Here's how the part is built. I have some questions about the finished solid (model axes, mm). A direction names the side the tool comes from. Give positions to 0.01 mm unless a question says otherwise; leave off trailing zeros. Write each loop counter-clockwise with the first axis right and the second up, starting at its lowest first coordinate (ties: lowest second). Pieces come first, ordered by that corner, then holes. Notation, with made-up numbers: (21.5, -24) -> (61.5, -24) arc R15 ccw to (61.5, -5) -> close; hole circle Ø10 at (56, 9.25). An arc over 180 degrees is marked (long way). Answer as CSV lines item,"result". Start each with the question number.
from build123d import *

# Parameters (mm, degrees)
BOX001_W     = 38.1
BOX001_H     = 12.7
BOX001_DEPTH = 50.8
BOX002_W     = 41.3004
BOX002_H     = 15.9004
BOX002_DEPTH = 50.8


with BuildPart() as cube001:
    # Box001 → Box001 (new body)
    with BuildSketch(Plane(origin=(1.6002, 1.6002, 1.6002), x_dir=(1, 0, 0), z_dir=(0, 0, 1))):
        with Locations((19.05, 6.35)):
            Rectangle(BOX001_W, BOX001_H)
    extrude(amount=BOX001_DEPTH)


with BuildPart() as cut:
    # Box002 → Box002 (new body)
    with BuildSketch(Plane.XY):
        with Locations((20.6502, 7.9502)):
            Rectangle(BOX002_W, BOX002_H)
    extrude(amount=BOX002_DEPTH)

    # Cut: cut Cube001
    add(cube001.part, mode=Mode.SUBTRACT)


with BuildPart() as cut_1:
    # Cut placement: moved
    add(cut.part.moved(Location((-15.8242, -7.874, -1.6002))))


solid = cut_1.part
Item 1: I'm going to push a flat-ended pin straight in: pin 1 (5 mm diameter, centred on x = 6.5, y = 0.5, fed in from +Z). Where does the tip first touch, or does it pass through?
Item 2: For faces 1 (the face through (5, 6.426, 24)), 2 (the face through (5, 7, 49.2)), which set-ups out of +Z, -Z, +X, -X, +Y, -Y let a thin tool reach every point of the face, with its end or its side?
Item 3: If we section it at C-C (x = 13.5): Please give me the cut outline in (y, z).
Item 4: If we section it at B-B (y = 3.5): Please give me the cut outline in (x, z).
Item 5: If I drill on line 1 (X direction, y = 4.75, z = 29); line 2 (Y direction, x = 9.5, z = 41); line 3 (Z direction, x = 21.5, y = -3.5), over which ranges is the centre line in solid material (lowest first)? Write a range as [from, to].
Item 6: We'd pull the mould along X, two halves only. Please class faces 3 (the face through (5, -6.274, 24)), 4 (the face through (5, -7.874, 23)), 5 (the face through (25.476, 0, 23)), 6 (the face through (-15.824, 0, 23)): released by +X, released by -X, zero draft, split by the parting line, or undercut.
Item 7: If we section it at A-A (z = 8.5): Please give me the cut outline in (x, y), and give its area (3 significant figures).
Final values:
1,pin 1,"z = 0"
2,face 1,"+Z"
2,face 2,"+Z, +X, -X, +Y, -Y"
3,outline,"(-7.87, -1.6) -> (8.03, -1.6) -> (8.03, 49.2) -> (6.43, 49.2) -> (6.43, 0) -> (-6.27, 0) -> (-6.27, 49.2) -> (-7.87, 49.2) -> close"
4,outline,"(-15.82, -1.6) -> (25.48, -1.6) -> (25.48, 49.2) -> (23.88, 49.2) -> (23.88, 0) -> (-14.22, 0) -> (-14.22, 49.2) -> (-15.82, 49.2) -> close"
5,line 1,"[-15.82, -14.22], [23.88, 25.48]"
5,line 2,"[-7.87, -6.27], [6.43, 8.03]"
5,line 3,"[-1.6, 0]"
6,face 3,"undercut"
6,face 4,"zero draft"
6,face 5,"released by +X"
6,face 6,"released by -X"
7,outline,"(-15.82, -7.87) -> (25.48, -7.87) -> (25.48, 8.03) -> (-15.82, 8.03) -> close; hole (-14.22, -6.27) -> (23.88, -6.27) -> (23.88, 6.43) -> (-14.22, 6.43) -> close"
7,area,"173 mm2"
